Source: CAD feature listing. Evaluate the final solid. Frame: model axes, mm. Face numbers are marked on the shaded views. A direction names the side the tool comes from. Round coordinates to 2 decimals unless told otherwise and drop trailing zeros. Order: outer loops, then holes, each group sorted by start corner. A loop starts at its lowest first (then second) coordinate and runs counter-clockwise, first axis right, second up. Notation, with made-up numbers: (56.5, 25.25) -> (114.5, 25.25) arc R17 ccw to (114.5, 30.25) -> close; hole circle Ø7 at (-4.75, -1.75). An arc over 180 degrees is marked (long way). One line per item, written item: value. Start each with the question number.
1) Section A-A (z = 27.5). Return the cut outline in (x, y).
2) Ray query, L1, parallel to Y at x = 101.9, z = 18.75; L2, parallel to X at y = 10.75, z = 16.75; L3, parallel to X at y = 8.75, z = 14.5. Return the intervals inside material, ascending.
3) Section B-B (x = 109.75). Return the cut outline in (y, z), and give its area (3 significant figures).
4) Pin query (flat end, axial travel): P1, Ø2.5, axis at x = 120, z = 31, coming from the +Y side; P2, Ø2, axis at x = 115.5, z = 13.5, coming from the +Y side; P3, Ø7, axis at x = 119.5, z = 29, coming from the -Y side. Return the tip coordinate at first contact, or that it passes through.
5) Section C-C (z = 18.75). Return the cut outline in (x, y), and give its area (3 significant figures).
6) Section D-D (y = 8.25). Return the cut outline in (x, z).
7) Reachability of the marked faces 1, 2 and 3 from +Z, -Z, +X, -X, +Y, -Y: full face, straight path, thin tool, end or side. Return the list, or none.
8) Mould query, pull axis Y, two halves, no side actions, for the marked faces 4, 5, 6 and 7. Classes: pulls with the +Y half, pulls with the -Y half, needs draft (parallel to the pull), parting line crosses it, or undercut.
```python
from build123d import *

# Parameters (mm, degrees)
OBJ1_DEPTH       = 5.04
OBJ1_PITCH_ANGLE = 90
OBJ2_W          = 5.04
OBJ2_H          = 6.24386
OBJ2_DEPTH      = 6.65
OBJ3_R          = 2.95
OBJ3_DEPTH      = 8.5
OBJ4         = 1.7
OBJ5     = 25
OBJ6     = -90
OBJ7_W                       = 12
OBJ7_H                       = 4
OBJ7_DEPTH                   = 9
GT2CLAMP0_CYL_R                       = 4
GT2CLAMP0_CYL_DEPTH                   = 9
OBJ8_DEPTH              = 23
OBJ9                       = 12
OBJ10                       = 4
OBJ11                   = 9


with BuildPart() as obj1:
    # obj1 → obj1 (new body)
    with BuildSketch(Plane.XY):
        Polygon((3.605, 0), (1.8025, 3.122022), (-1.8025, 3.122022), (-3.605, 0), (-1.8025, -3.122022), (1.8025, -3.122022), align=None)
    extrude(amount=OBJ1_DEPTH)


with BuildPart() as obj1_1:
    # obj1 pitch: moved
    add(obj1.part.rotate(Axis((0, 0, 0), (0, 1, 0)), OBJ1_PITCH_ANGLE))


with BuildPart() as obj1_2:
    # obj1 placement: moved
    add(obj1_1.part.moved(Location((3, 8.004167, 6.65))))


with BuildPart() as obj2:
    # obj2 → obj2 (new body)
    with BuildSketch(Plane(origin=(3, 4.882237, 0), x_dir=(1, 0, 0), z_dir=(0, 0, 1))):
        with Locations((2.52, 3.12193)):
            Rectangle(OBJ2_W, OBJ2_H)
    extrude(amount=OBJ2_DEPTH)


with BuildPart() as obj3:
    # obj3 → obj3 (new body)
    with BuildSketch(Plane.XY.offset(-1)):
        Circle(OBJ3_R)
    extrude(amount=OBJ3_DEPTH)


with BuildPart() as gt2clamp0_clamp_hole:
    with BuildSketch(Plane.XY.offset(-1)):
        Circle(OBJ4)
    extrude(amount=OBJ5)

    add(obj3.part)


with BuildPart() as gt2clamp0_clamp_hole_1:
    add(gt2clamp0_clamp_hole.part.rotate(Axis((0, 0, 0), (0, 1, 0)), OBJ6))


with BuildPart() as gt2clamp0_clamp_hole_2:
    add(gt2clamp0_clamp_hole_1.part.moved(Location((23, 8.004167, 6.25))))

    # gt2clamp0_clamp_hole: union obj1, obj2
    add(obj1_2.part)
    add(obj2.part)


with BuildPart() as obj7:
    # obj7 → obj7 (new body)
    with BuildSketch(Plane(origin=(11, 9.404167, 11.5), x_dir=(1, 0, 0), z_dir=(0, 0, 1))):
        with Locations((6, 2)):
            Rectangle(OBJ7_W, OBJ7_H)
    extrude(amount=OBJ7_DEPTH)


with BuildPart() as gt2clamp0_cyl:
    # gt2clamp0_cyl → gt2clamp0_cyl (new body)
    with BuildSketch(Plane(origin=(4, 8.004167, 11.5), x_dir=(1, 0, 0), z_dir=(0, 0, 1))):
        Circle(GT2CLAMP0_CYL_R)
    extrude(amount=GT2CLAMP0_CYL_DEPTH)


with BuildPart() as obj8:
    # gt2clamp0base_plane_yz → obj8 (new body)
    with BuildSketch(Plane(origin=(0, 8.004167, 6.25), x_dir=(0, 1, 0), z_dir=(-1, 0, 0))):
        Polygon((-5.2, 6.25), (-5.2, 3.50625), (-7.804167, 0.902083), (-7.804167, -0.902083), (-5.2, -3.50625), (-5.2, -6.25), (5.2, -6.25), (5.2, -3.50625), (7.804167, -0.902083), (7.804167, 0.902083), (5.2, 3.50625), (5.2, 6.25), align=None)
    extrude(amount=-OBJ8_DEPTH)


with BuildPart() as gt2clamp0:
    with BuildSketch(Plane(origin=(11, 2.604167, 11.5), x_dir=(1, 0, 0), z_dir=(0, 0, 1))):
        with Locations((6, 2)):
            Rectangle(OBJ9, OBJ10)
    extrude(amount=OBJ11)

    # gt2clamp0clamp_base: union obj7, gt2clamp0_cyl, obj8
    add(obj7.part)
    add(gt2clamp0_cyl.part)
    add(obj8.part)

    # gt2clamp0: cut gt2clamp0_clamp_hole
    add(gt2clamp0_clamp_hole_2.part, mode=Mode.SUBTRACT)


with BuildPart() as gt2clamp0_1:
    # gt2clamp0 placement: moved
    add(gt2clamp0.part.moved(Location((100, 1.2, 12.5))))


solid = gt2clamp0_1.part
```
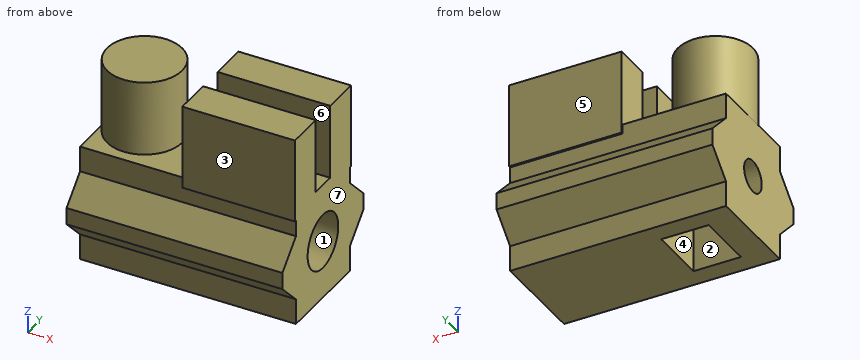
Findings:
1. outline: circle Ø8 at (104, 9.2); (111, 3.8) -> (123, 3.8) -> (123, 7.8) -> (111, 7.8) -> close; (111, 10.6) -> (123, 10.6) -> (123, 14.6) -> (111, 14.6) -> close
2. L1: 1.4 to 7.5, 10.9 to 17.01
2. L2: 100 to 103, 108.04 to 115.5
2. L3: 100 to 103, 108.04 to 123
3. outline: (1.4, 17.85) -> (4, 15.24) -> (4, 12.5) -> (14.4, 12.5) -> (14.4, 15.24) -> (17.01, 17.85) -> (17.01, 19.65) -> (14.4, 22.26) -> (14.4, 25) -> (4, 25) -> (4, 22.26) -> (1.4, 19.65) -> close; hole circle Ø3.4 at (9.2, 18.75)
3. area: 144 mm2
4. P1: y = 14.6
4. P2: y = 14.4
4. P3: y = 3.8
5. outline: (100, 1.4) -> (123, 1.4) -> (123, 6.25) -> (115.5, 6.25) -> (115.5, 7.5) -> (108.04, 7.5) -> (108.04, 6.08) -> (103, 6.08) -> (103, 7.5) -> (100, 7.5) -> close; (100, 10.9) -> (103, 10.9) -> (103, 12.33) -> (108.04, 12.33) -> (108.04, 10.9) -> (115.5, 10.9) -> (115.5, 12.15) -> (123, 12.15) -> (123, 17.01) -> (100, 17.01) -> close
5. area: 248 mm2
6. outline: (100, 12.5) -> (103, 12.5) -> (103, 17.34) -> (100, 17.34) -> close; (100, 20.16) -> (103, 20.16) -> (103, 22.2) -> (108.04, 22.2) -> (108.04, 20.16) -> (115.5, 20.16) -> (115.5, 21.54) -> (123, 21.54) -> (123, 25) -> (107.88, 25) -> (107.88, 33) -> (100.12, 33) -> (100.12, 25) -> (100, 25) -> close; (108.04, 12.5) -> (123, 12.5) -> (123, 15.96) -> (115.5, 15.96) -> (115.5, 17.34) -> (108.04, 17.34) -> close
7. face 1: +X
7. face 2: -Z
7. face 3: +Z, +X, -X, -Y
8. face 4: undercut
8. face 5: pulls with the +Y half
8. face 6: undercut
8. face 7: needs draft
